For this review, take the finished solid that the model builds, in its own axes (mm). Give positions to 0.01 mm unless a question says otherwise; leave off trailing zeros. Order: outer loops, then holes, each group sorted by start corner. A loop starts at its lowest first (then second) coordinate and runs counter-clockwise, first axis right, second up. Notation, with made-up numbers: (56, 10) - (68, 10) arc R37 ccw to (68, 47) - close; hole circle Ø6 at (-26.75, -36). An arc over 180 degrees is marked (long way). One line per item, written item: value.
```python
from build123d import *

# Parameters (mm, degrees)
SKETCH1_W           = 105
SKETCH1_H           = 12.3
BOSS_EXTRUDE1_DEPTH = 5
SKETCH2_W           = 5
SKETCH2_H           = 5
BOSS_EXTRUDE2_DEPTH = 5
SKETCH3_W           = 73
SKETCH3_H           = 5
CUT_EXTRUDE1_DEPTH  = 17
SKETCH4_W           = 5
SKETCH4_H           = 5
BOSS_EXTRUDE3_DEPTH = 5


with BuildPart() as part:
    # Sketch1 → Boss-Extrude1 (new body)
    with BuildSketch(Plane.XY):
        Rectangle(SKETCH1_W, SKETCH1_H)
    extrude(amount=BOSS_EXTRUDE1_DEPTH)

    # Sketch2 → Boss-Extrude2 (add)
    with BuildSketch(Plane.XZ.offset(6.15)):
        with Locations((-50, 2.5)):
            Rectangle(SKETCH2_W, SKETCH2_H)
        with Locations((50, 2.5)):
            Rectangle(SKETCH2_W, SKETCH2_H)
    extrude(amount=BOSS_EXTRUDE2_DEPTH)

    # Mirror1: part across plane


with BuildPart() as part_1:
    add(part.part)
    add(part.part.mirror(Plane(origin=(-52.5, 6.15, 5), x_dir=(0, 0, 1), z_dir=(0, -1, 0))))

    # Sketch3 → Cut-Extrude1 (cut)
    with BuildSketch(Plane(origin=(0, 18.45, 0), x_dir=(1, 0, 0), z_dir=(0, 1, 0))):
        with Locations((6.5, -2.5)):
            Rectangle(SKETCH3_W, SKETCH3_H)
    extrude(amount=-CUT_EXTRUDE1_DEPTH, mode=Mode.SUBTRACT)

    # Sketch4 → Boss-Extrude3 (add)
    with BuildSketch(Plane.XZ.offset(6.15)):
        with Locations((0, 2.5)):
            Rectangle(SKETCH4_W, SKETCH4_H)
    extrude(amount=BOSS_EXTRUDE3_DEPTH)


solid = part_1.part
```
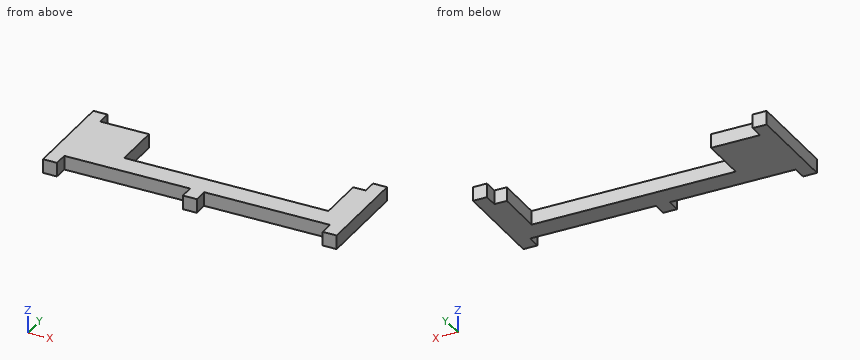
(1) Take a section at B-B (z = 3.25). Write out the cut boundary in (x, y), then the cut area to 3 significant figures.
Answers below:
outline: (-52.5, -11.15) - (-47.5, -11.15) - (-47.5, -6.15) - (-2.5, -6.15) - (-2.5, -11.15) - (2.5, -11.15) - (2.5, -6.15) - (47.5, -6.15) - (47.5, -11.15) - (52.5, -11.15) - (52.5, 23.45) - (47.5, 23.45) - (47.5, 18.45) - (43, 18.45) - (43, 1.45) - (-30, 1.45) - (-30, 18.45) - (-47.5, 18.45) - (-47.5, 23.45) - (-52.5, 23.45) - close
area: 1,470 mm^2
(2) For P1, Ø2.5, axis at x = -37, z = 3, coming from the +Y side; P2, Ø1, axis at x = 15.5, z = 2, coming from the -Y side; P3, Ø3, axis at x = 19, y = 2.5, coming from the -Z side; P4, Ø3, axis at x = -15.5, z = 2.5, coming from the +Y side, all flat-tipped, find the tip position at first contact; note any pin that passes through.
Answers below:
P1: stops at y = 18.45
P2: stops at y = -6.15
P3: stops at z = 0
P4: stops at y = 1.45
(3) Take a section at A-A (y = 3.5). Write out the cut boundary in (x, z).
Answers below:
outline: (-52.5, 0) - (-30, 0) - (-30, 5) - (-52.5, 5) - close; (43, 0) - (52.5, 0) - (52.5, 5) - (43, 5) - close
(4) Take a section at C-C (x = -11.5). Write out the cut boundary in (y, z), then the cut area to 3 significant figures.
Answers below:
outline: (-6.15, 0) - (1.45, 0) - (1.45, 5) - (-6.15, 5) - close
area: 38.0 mm^2
(5) Wall thickness on line 1 (X direction, y = 3, z = 3.65); line 2 (Y direction, x = -35, z = 1.6); line 3 (X direction, y = 20.5, z = 2.2): over which ranges is each line inside the solid? List them lowest first. Write a range as from..to.
Answers below:
line 1: x = -52.5..-30, 43..52.5
line 2: y = -6.15..18.45
line 3: x = -52.5..-47.5, 47.5..52.5
